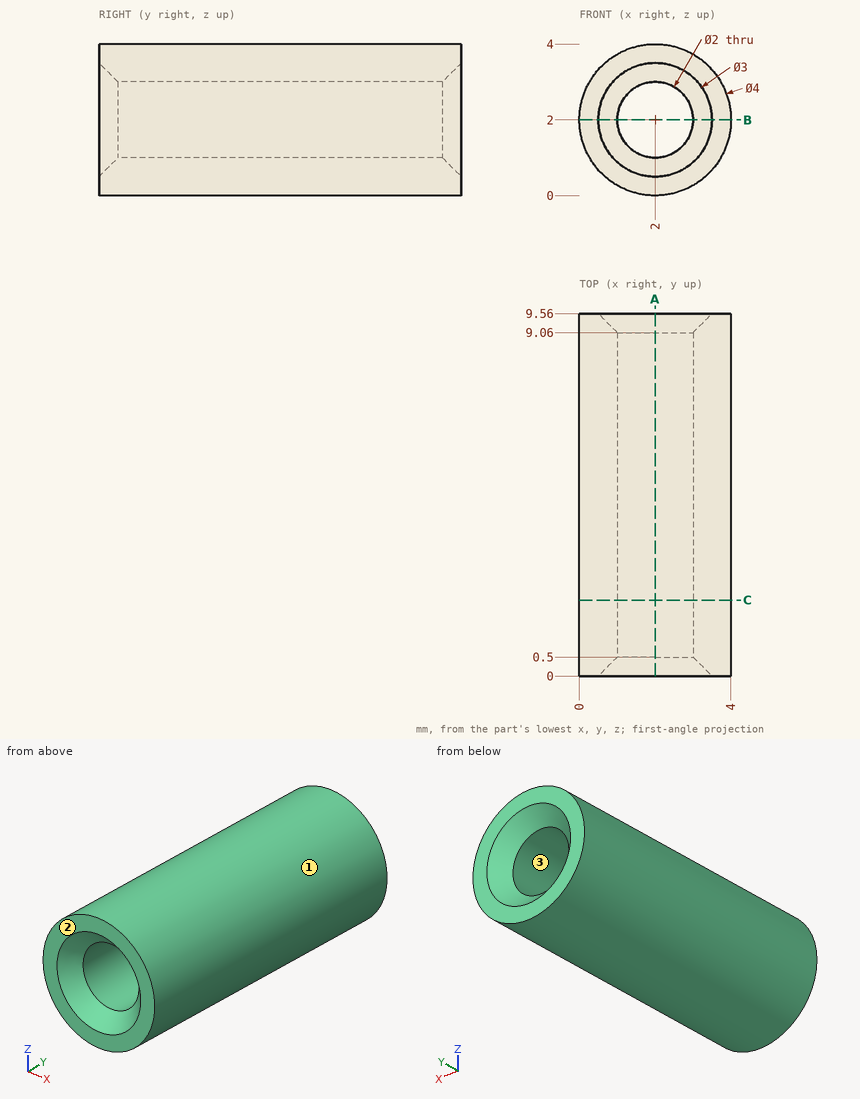
Job drawing, mm, ordinate dimensions from the low corner. One solid piece. Coordinates: 2 decimals unless noted, no trailing zeros. Loops run counter-clockwise (first coordinate to the right, second up) from the corner with the lowest first, then second, coordinate; pieces in that order, holes last. Notation, with made-up numbers: (56.25, -12.75) -> (114.25, -12.75) arc R13 cw to (114.25, 2.25) -> close; hole circle Ø11 at (-22, 3.25). An arc over 180 degrees is marked (long way). One line per item, written item: value.
1. Slice it at B-B on z = 2. Write the cut outline in (x, y), and give its area (3 significant figures).
Answers:
outline: (0, 0) -> (0.5, 0) -> (1, 0.5) -> (1, 9.06) -> (0.5, 9.56) -> (0, 9.56) -> close; (3, 0.5) -> (3.5, 0) -> (4, 0) -> (4, 9.56) -> (3.5, 9.56) -> (3, 9.06) -> close
area: 18.6 mm^2
2. Pull direction X, two halves, no side cores. Call the marked faces 1, 2 and 3: pulls with the +X half, pulls with the -X half, needs draft (parallel to the pull), parting line crosses it, or undercut.
Answers:
face 1: parting line crosses it
face 2: needs draft
face 3: undercut
3. Drill centre lines: line 1 (Z direction, x = 2, y = 3.5); line 2 (X direction, y = 2.75, z = 1.65); line 3 (Z direction, x = 2.4, y = 4). Where is each one in solid material? Low to high. Write a range as [from, to].
Answers:
line 1: z = [0, 1], [3, 4]
line 2: x = [0.03, 1.06], [2.94, 3.97]
line 3: z = [0.04, 1.08], [2.92, 3.96]
4. Flat gauge pins, fed straight in: P1, Ø1, axis at x = 3.5, y = 8, coming from the -Z side; P2, Ø2, axis at x = 1, z = 1, coming from the +Y side; P3, Ø1, axis at y = 5.5, z = 1, coming from the -X side. Where does each tip first touch, or does it go through?
Answers:
P1: stops at z = 0.27
P2: stops at y = 9.56
P3: stops at x = 0.06
5. Slice it at A-A on x = 2. Write the cut outline in (y, z).
Answers:
outline: (0, 0) -> (9.56, 0) -> (9.56, 0.5) -> (9.06, 1) -> (0.5, 1) -> (0, 0.5) -> close; (0, 3.5) -> (0.5, 3) -> (9.06, 3) -> (9.56, 3.5) -> (9.56, 4) -> (0, 4) -> close
6. Slice it at C-C on y = 2. Write the cut outline in (x, z), and give its area (3 significant figures).
Answers:
outline: circle Ø4 at (2, 2); hole circle Ø2 at (2, 2)
area: 9.42 mm^2
